CAD build for the part. Positions are in the model's coordinates, mm. A direction names the side the tool comes from. Round coordinates to 2 decimals unless told otherwise and drop trailing zeros. Order: outer loops, then holes, each group sorted by start corner. A loop starts at its lowest first (then second) coordinate and runs counter-clockwise, first axis right, second up. Notation, with made-up numbers: (-2.75, 50.5) -> (23.25, 50.5) arc R34 ccw to (23.25, 88.5) -> close; hole circle Ø9 at (63.5, 79). An arc over 180 degrees is marked (long way). Return JSON: item names as keys, results as strings. Group by question number.
Q1. Probe line 1 along X through (y, z) = (2, 0); line 2 along Y through (x, z) = (5.5, -1.25); line 3 along X through (y, z) = (1.4, -2.25). List the from-to ranges inside material, lowest first.
Q2. Flat gauge pins, fed straight in: pin 1 (1 mm diameter, centred on x = 2.5, y = 1.5, fed in from +Z); pin 2 (1.1 mm diameter, centred on x = 0, z = -6.5, fed in from -Y); pin 3 (5.5 mm diameter, centred on x = 1, z = 0, fed in from -Y); pin 4 (1.5 mm diameter, centred on y = 3.5, z = 6.5, fed in from -X). Where does each tip first touch, or does it go through?
Q3. Which spindle directions (+Z, -Z, +X, -X, +Y, -Y) get a long thin tool onto all of the face, cutting with end or side? Do faces 1 (the flat face through (0, 4.7, 0)), 2 (the flat face through (0, 3, 0)). Say none if no direction does.
Q4. Cut at B-B (z = 3.25). Write the cut outline in (x, y), then the cut area to 3 significant figures.
Q5. Mould opens along X. For faces 3 (the cylindrical face through (-2.44, 1.48, -0.54)), 4 (the flat face through (0, 3, 6)) say: +X half, -X half, draft (parallel to the pull), parting line (faces both ways), or undercut.
Q6. Cut at C-C (x = 2.75). Write the cut outline in (y, z), then the cut area to 3 significant figures.
Q7. Cut at A-A (y = 0.65). Write the cut outline in (x, z), then the cut area to 3 significant figures.
from build123d import *

# Parameters (mm, degrees)
SKETCH_1_R      = 4
SKETCH_1_R_2    = 2.5
EXTRUDE_1_DEPTH = 3
SKETCH_2_R      = 4
EXTRUDE_2_DEPTH = 1.7


with BuildPart() as part:
    # 草图1 → 凸台-拉伸1 (new body)
    with BuildSketch(Plane(origin=(0, 0, 0), x_dir=(1, 0, 0), z_dir=(0, 1, 0))):
        with Locations(Location((0, 0, 0), (0, 0, 270))):
            Circle(SKETCH_1_R)
        with Locations(Location((0, 0, 0), (0, 0, 270))):
            Circle(SKETCH_1_R_2, mode=Mode.SUBTRACT)
    extrude(amount=EXTRUDE_1_DEPTH)

    # 草图2 → 凸台-拉伸2 (add)
    with BuildSketch(Plane(origin=(0, 3, 0), x_dir=(1, 0, 0), z_dir=(0, 1, 0))):
        with BuildLine():
            ThreePointArc((3.601811154, 1.73981505), (3.899182261, 0.892399962), (4, 0))
            ThreePointArc((4, 0), (3.873348744, -0.998583752), (3.501415245, -1.933931561))
            add(Edge.make_bspline(
                [(3.501415245, -1.933931561), (22.78951803, -0.622790472), (3.601811154, 1.73981505)],
                knots=[1.976614939, 1.976614939, 1.976614939, 4.306570368, 4.306570368, 4.306570368], degree=2, weights=[1, 0.394771017, 1]))
        make_face()
        with BuildLine():
            ThreePointArc((-1.73981505, 3.601811154), (0.109270946, 3.998507204), (1.933931561, 3.501415245))
            add(Edge.make_bspline(
                [(1.933931561, 3.501415245), (0.622790472, 22.78951803), (-1.73981505, 3.601811154)],
                knots=[5.118207593, 5.118207593, 5.118207593, 7.448163021, 7.448163021, 7.448163021], degree=2, weights=[1, 0.394771017, 1]))
        make_face()
        with BuildLine():
            ThreePointArc((-3.601811154, -1.73981505), (-3.998507204, 0.109270946), (-3.501415245, 1.933931561))
            add(Edge.make_bspline(
                [(-3.501415245, 1.933931561), (-22.78951803, 0.622790472), (-3.601811154, -1.73981505)],
                knots=[5.118207593, 5.118207593, 5.118207593, 7.448163021, 7.448163021, 7.448163021], degree=2, weights=[1, 0.394771017, 1]))
        make_face()
        with BuildLine():
            add(Edge.make_bspline(
                [(-1.933931561, -3.501415245), (-0.622790472, -22.78951803), (1.73981505, -3.601811154)],
                knots=[1.976614939, 1.976614939, 1.976614939, 4.306570368, 4.306570368, 4.306570368], degree=2, weights=[1, 0.394771017, 1]))
            ThreePointArc((1.73981505, -3.601811154), (-0.109270946, -3.998507204), (-1.933931561, -3.501415245))
        make_face()
        with Locations(Location((0, 0, 0), (0, 0, 115.782351759))):
            Circle(SKETCH_2_R)
    extrude(amount=EXTRUDE_2_DEPTH)


solid = part.part
Solution:
{
 "1": {"line 1": "x = -4 to -2.5, 2.5 to 4", "line 2": "y = 3 to 4.7", "line 3": "x = -3.31 to -1.09, 1.09 to 3.31"},
 "2": {"pin 1": "stops at z = 3.46", "pin 2": "stops at y = 3", "pin 3": "stops at y = 0", "pin 4": "stops at x = -1.69"},
 "3": {"face 1": "+Z, -Z, +X, -X, +Y", "face 2": "-Y"},
 "4": {"outline": "(-2.33, 0) -> (2.33, 0) -> (2.33, 4.7) -> (-2.33, 4.7) -> close", "area": "21.9 mm²"},
 "5": {"face 3": "undercut", "face 4": "draft"},
 "6": {"outline": "(0, -2.9) -> (4.7, -2.9) -> (4.7, 2.9) -> (0, 2.9) -> close", "area": "27.3 mm²"},
 "7": {"outline": "circle Ø8 at (0, 0); hole circle Ø5 at (0, 0)", "area": "30.6 mm²"}
}
